For this review, take the finished solid that the model builds, in its own axes (mm). Face numbers are marked on the shaded views. A direction names the side the tool comes from. Coordinates: 2 decimals unless noted, no trailing zeros. Write each loop counter-clockwise with the first axis right and the second up, starting at its lowest first coordinate (ties: lowest second). Pieces come first, ordered by that corner, then holes.
Solid Edge part; units mm, degrees
sketch "Sketch1" plane through (0, 0, 0) normal (1, 0, 0) x (0, 1, 0)
  line L0 (0, 11.5) -> (2.3, 11.5)
  line L1 (2.3, 11.5) -> (4.7847, 11.0619)
  arc A0 (4.7847, 11.0619) -> (4.95, 10.8649) centre (4.75, 10.8649) cw
  line L2 (4.95, 10.8649) -> (4.95, 10)
  line L3 (4.95, 10) -> (2.7, 10)
  arc A1 (2.7, 10) -> (2.4, 9.7) centre (2.7, 9.7) ccw
  line L4 (2.4, 9.7) -> (2.4, 9)
  line L5 (2.4, 9) -> (3.75, 9)
  line L6 (3.75, 9) -> (3.95, 8.8)
  line L7 (3.95, 8.8) -> (3.95, 8.1)
  line L8 (3.95, 8.1) -> (3.85, 8)
  line L9 (3.85, 8) -> (3.95, 7.9)
  line L10 (3.95, 7.9) -> (3.95, 5.9)
  line L11 (3.95, 5.9) -> (8.4, 5.9)
  line L12 (8.4, 5.9) -> (8.4, 2.4249)
  line L13 (8.4, 2.4249) -> (7, 0)
  line L14 (7, 0) -> (0, 0)
  line L15 (0, 0) -> (0, 11.5)
revolve "RevolvedProtrusion1" add sketch "Sketch1" angle 360 about axis through (0, 0, 0) along (0, 0, 1)
sketch "Sketch2" plane through (0, 0, 0) normal (0, 0, 1) x (1, 0, 0)
  line L0 (-14, -14) -> (14, -14)
  line L1 (14, -14) -> (14, 14)
  line L2 (14, 14) -> (-14, 14)
  line L3 (-14, 14) -> (-14, -14)
  line L4 (-7, -4.0415) -> (0, -8.0829)
  line L5 (0, -8.0829) -> (7, -4.0415)
  line L6 (7, -4.0415) -> (7, 4.0415)
  line L7 (7, 4.0415) -> (0, 8.0829)
  line L8 (0, 8.0829) -> (-7, 4.0415)
  line L9 (-7, 4.0415) -> (-7, -4.0415)
extrude "Cutout1" cut sketch "Sketch2" along normal blind 6
sketch "Sketch3" plane through (0, 0, 0) normal (1, 0, 0) x (0, 1, 0)
  line L0 (4.35, 5.9) -> (4.6964, 5.3)
  line L1 (4.6964, 5.3) -> (4.85, 5.3)
  line L2 (4.85, 5.3) -> (4.85, 4.9)
  line L3 (4.85, 4.9) -> (14.85, 2.2205)
  line L4 (14.85, 2.2205) -> (14.85, 5.9)
  line L5 (14.85, 5.9) -> (4.35, 5.9)
revolve "RevolvedCutout1" cut sketch "Sketch3" angle 360 about axis through (0, 0, -50) along (0, 0, 1)
sketch "Sketch4" plane through (0, 0, 0) normal (1, 0, 0) x (0, 1, 0)
  line L0 (0, 0) -> (6.7346, 0)
  line L1 (6.7346, 0) -> (6.4188, -10.1164)
  line L2 (6.4188, -10.1164) -> (5.5352, -11)
  line L3 (5.5352, -11) -> (0, -11)
  line L4 (0, -11) -> (0, 0)
revolve "RevolvedProtrusion2" add sketch "Sketch4" angle 360 about axis through (0, 0, -11) along (0, 0, 1)
sketch "Sketch5" plane through (0, 0, 0) normal (1, 0, 0) x (0, 1, 0)
  line L0 (0, 11.5) -> (2.3, 11.5)
  arc A0 (2.3, 11.5) -> (2, 11.2) centre (2.3, 11.2) ccw
  line L1 (2, 11.2) -> (2, -3.4)
  line L2 (2, -3.4) -> (1.5, -3.4)
  line L3 (1.5, -3.4) -> (1.5, -5.1017)
  line L4 (1.5, -5.1017) -> (3.7591, -5.5)
  line L5 (3.7591, -5.5) -> (3.7591, -10.5)
  line L6 (3.7591, -10.5) -> (4.2591, -11)
  line L7 (4.2591, -11) -> (0, -11)
  line L8 (0, -11) -> (0, 11.5)
revolve "RevolvedCutout2" cut sketch "Sketch5" angle 360 about axis through (0, 0, -11) along (0, 0, 1)
properties part number "190644 QS-1/4-4"
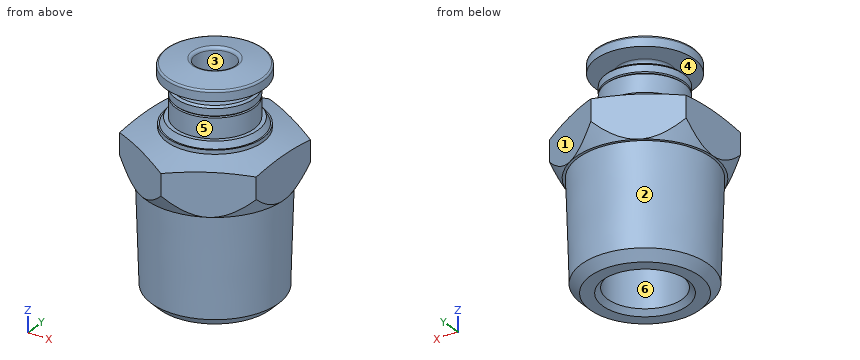
Q1. Add section A-A (z = 1). State the section outline as (x, y) points, then the cut area to 3 significant figures.
Ans:
outline: (-7, -2.9) arc R7.58 ccw to (-6.01, -4.61) - (-0.99, -7.51) arc R7.58 ccw to (0.99, -7.51) - (6.01, -4.61) arc R7.58 ccw to (7, -2.9) - (7, 2.9) arc R7.58 ccw to (6.01, 4.61) - (0.99, 7.51) arc R7.58 ccw to (-0.99, 7.51) - (-6.01, 4.61) arc R7.58 ccw to (-7, 2.9) - close; hole circle Ø4 at (0, 0)
area: 154 mm2
Q2. Clearance check with flat-ended pins moving along their axes: pin 1 Ø8 at (x, z) = (-5, 4.5) entering from +Y; pin 2 Ø4.5 at (x, y) = (0, 0) entering from -Z; pin 3 Ø5 at (y, z) = (-1.5, -6.5) entering from +X. State where each tip first meets the part, or that it passes through.
Ans:
pin 1: stops at y = 7.5
pin 2: stops at z = -5.23
pin 3: stops at x = 6.6
Q3. Add section B-B (z = 7). State the section outline as (x, y) points, then the cut area to 3 significant figures.
Ans:
outline: circle Ø7.9 at (0, 0); hole circle Ø4 at (0, 0)
area: 36.5 mm2
Q4. Tool access review of the marked faces 1 and 2: name each direction out of +Z, -Z, +X, -X, +Y, -Y from which nothing blocks a thin tool from reaching the whole face with its end or side.
Ans:
face 1: +Z, -Z, +X, +Y
face 2: -Z
Q5. Add section C-C (z = -8.25). State the section outline as (x, y) points.
Ans:
outline: circle Ø12.95 at (0, 0); hole circle Ø7.52 at (0, 0)
Q6. Draft analysis for pull direction X (two halves, no side actions). For the marked faces 3, 4, 5 and 6, state which applies: +X half, -X half, draft (parallel to the pull), parting line (faces both ways), or undercut.
Ans:
face 3: undercut
face 4: draft
face 5: parting line
face 6: undercut
Q7. For probe 1 along Y at (x, z) = (0, 5); probe 2 along Z at (x, y) = (4.25, 2.75); probe 3 along X at (y, z) = (-1, 1.5), list the stretches that pass through material, from the lowest coordinate up.
Ans:
probe 1: y = -4.85 to -2, 2 to 4.85
probe 2: z = -11 to 4.84
probe 3: x = -7 to -1.73, 1.73 to 7
